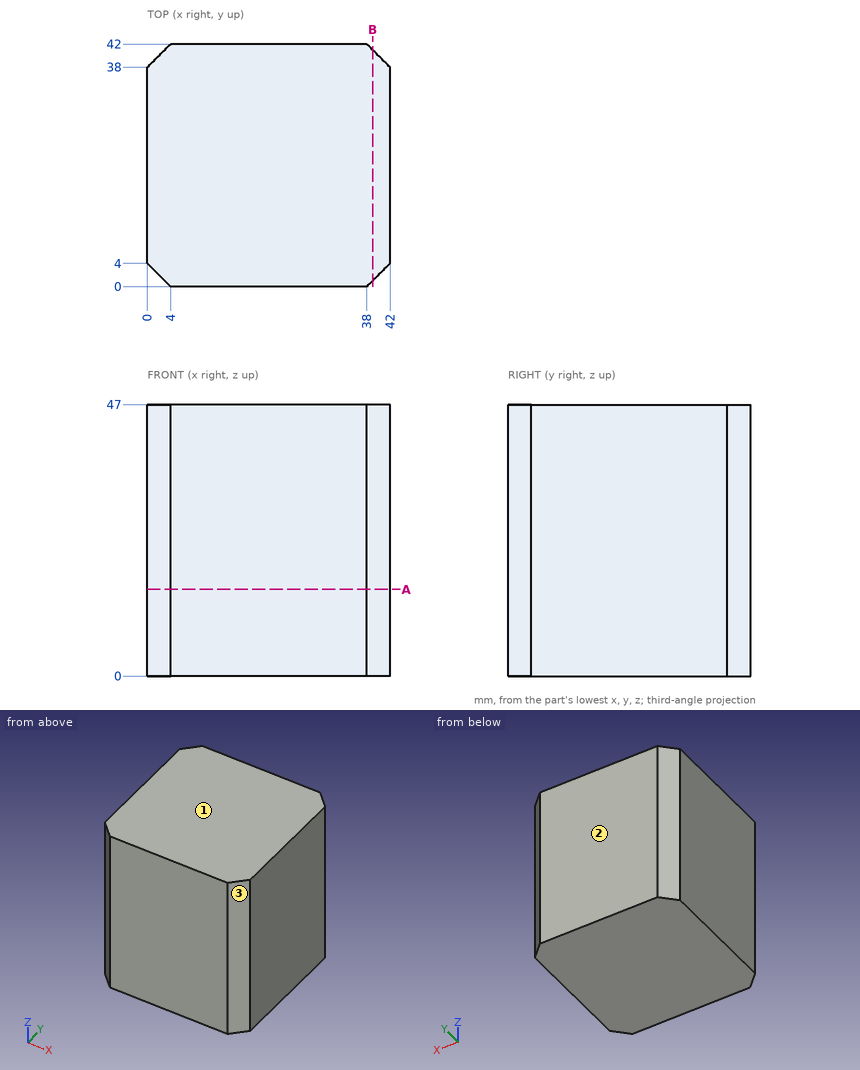
Answer from the drawing. Dimensions are ordinates in mm from the lowest x, y and z of the part. Coordinates: 2 decimals unless noted, no trailing zeros. Loops run counter-clockwise (first coordinate to the right, second up) from the corner with the lowest first, then second, coordinate; pieces in that order, holes last. Notation, with made-up numbers: (-7.75, 1.25) -> (4.25, 1.25) arc R27 cw to (4.25, 40.25) -> close; hole circle Ø1 at (-27, -6.75). An arc over 180 degrees is marked (long way). Return JSON: item names as keys, results as strings.
Item 1: A flat-ended cylindrical pin translates along its axis: P1, Ø10, axis at x = 31, z = 41, coming from the -Y side. Find the tip coordinate at first contact, or state that the pin passes through.
Answers:
{"P1": "stops at y = 0"}
Item 2: Find section A-A (z = 15). Determine the outline of the cut face in (x, y), plus the area to 3 significant figures.
Answers:
{"outline": "(0, 4) -> (4, 0) -> (38, 0) -> (42, 4) -> (42, 38) -> (38, 42) -> (4, 42) -> (0, 38) -> close", "area": "1,730 mm2"}
Item 3: Find the intervals of material crossed by probe 1 along Y at (x, z) = (40.5, 27); probe 2 along X at (y, z) = (40, 37), in increasing order.
Answers:
{"probe 1": "y = 2.5 to 39.5", "probe 2": "x = 2 to 40"}
Item 4: For a pull along Y with two mould halves and no side action, classify the marked faces 1, 2 and 3 as +Y half, -Y half, draft (parallel to the pull), parting line (faces both ways), or undercut.
Answers:
{"face 1": "draft", "face 2": "+Y half", "face 3": "-Y half"}
Item 5: Find section B-B (x = 39). Determine the outline of the cut face in (y, z).
Answers:
{"outline": "(1, 0) -> (41, 0) -> (41, 47) -> (1, 47) -> close"}
